Source: CAD feature listing. Evaluate the final solid. Frame: model axes, mm. A direction names the side the tool comes from. Coordinates: 2 decimals unless noted, no trailing zeros. Write each loop counter-clockwise with the first axis right and the second up, starting at its lowest first coordinate (ties: lowest second). Pieces come first, ordered by that corner, then holes. Notation, with made-up numbers: (-31, -22.75) - (-14, -22.75) arc R17 ccw to (-14, -6.75) - close; hole circle Ø11 at (28.5, -25.5). An arc over 180 degrees is marked (long way). One line per item, written item: value.
Autodesk Inventor part; units mm, degrees
ref_plane "YZ Plane" through (0, 0, 0) normal (1, 0, 0) x (0, 1, 0)
ref_plane "XZ Plane" through (0, 0, 0) normal (0, 1, 0) x (-1, 0, 0)
ref_plane "XY Plane" through (0, 0, 0) normal (0, 0, 1) x (1, 0, 0)
sketch "Sketch1" plane through (0, 0, 0) normal (0, 0, 1) x (1, 0, 0)
  arc A0 (6.1342, -1.6415) -> (-4.4197, 4.5595) centre (0, 0) ccw
  circle A1 centre (0, 0) radius 9.525 construction
  line L0 (3.175, -12.7) -> (-22.225, -12.7)
  line L1 (-22.225, -12.7) -> (-22.225, -63.5)
  line L2 (-22.225, -63.5) -> (3.175, -63.5)
  line L3 (3.175, -63.5) -> (3.175, -12.7)
  line L4 (3.175, -12.7) -> (-22.225, -63.5) construction
  line L5 (-22.225, -12.7) -> (3.175, -63.5) construction
  line L6 (9.525, 7.0623) -> (9.525, -12.9681) construction
  circle A2 centre (-9.525, -25.4) radius 2.4892
  circle A3 centre (-9.525, -38.1) radius 2.4892
  circle A4 centre (-9.525, -50.8) radius 2.4892
  circle A5 centre (0, 0) radius 2.3813
  line L7 (3.175, -12.7) -> (6.1342, -1.6415)
  line L8 (-4.4197, 4.5595) -> (-22.225, -12.7)
  line L9 (3.175, -63.5) -> (-22.225, -63.5)
  line L10 (-22.225, -63.5) -> (-22.225, -57.15)
  line L11 (-22.225, -57.15) -> (3.175, -57.15)
  line L12 (3.175, -57.15) -> (3.175, -63.5)
  line L13 (-22.225, -63.5) -> (-13.843, -63.5)
  line L14 (-13.843, -63.5) -> (-13.843, -44.45)
  line L15 (-13.843, -44.45) -> (-22.225, -44.45)
  line L16 (-22.225, -44.45) -> (-22.225, -63.5)
  point P0 (-13.843, -57.15)
  point P1 (3.175, -57.15)
  dimension "d0" = 12.7
  dimension "d1" = 19.05
  dimension "d2" = 25.4
  dimension "d4" = 6.35
  dimension "d5" = 4.9784
  dimension "d8" = 12.7
  dimension "d13" = 4.7625
  dimension "d17" = 3.175
  dimension "d18" = 12.7
  dimension "d19" = 6.35
  dimension "d20" = 8.382
  dimension "d21" = 19.05
extrude "Extrusion1" add sketch "Sketch1" along normal blind 3.175 contours L7 L0 L8 A0 | L3 L11 L14 L15 L1 L0 | L15 L14 L11 L1
fillet "Fillet1" radius 3.175 4 edges at (3.175, -12.7, 1.5875) (-22.225, -12.7, 1.5875) (3.175, -57.15, 1.5875) (-22.225, -57.15, 1.5875)
properties part number "Top Bearing Plate (R4 - 0.25in Between Stages)" material "Aluminum 6061"
1) Material intervals for line 1 (Y direction, x = 0, z = 1.7); line 2 (Y direction, x = -10, z = 0.75); line 3 (Y direction, x = -11, z = 2), sorted ascending.
Values found:
line 1: -57.15 to -2.38, 2.38 to 6.35
line 2: -57.15 to -53.24, -48.36 to -40.54, -35.66 to -27.84, -22.96 to -0.85
line 3: -57.15 to -52.81, -48.79 to -40.11, -36.09 to -27.41, -23.39 to -1.82
2) Contact query for flat-ended pins moving along their axis: P1, Ø4, axis at x = -9.525, y = -50.8, coming from the -Z side; P2, Ø1.6, axis at y = -23.5, z = 1, coming from the +X side (3 decimals). Output: stop coordinate, or through.
Values found:
P1: through
P2: x = 3.175
3) Draft query along Y for faces 3 (the cylindrical face through (2.22, -56.245, 1.61)), 4 (the flat face through (-5, -25, 0)), 5 (the cylindrical face through (-11.36, -27.08, 1.57)), 6 (the cylindrical face through (1.1, 2.11, 1.57)). Return one class per face: released by +Y, released by -Y, zero draft, split by the parting line, or undercut.
Values found:
face 3: released by -Y
face 4: zero draft
face 5: undercut
face 6: undercut
4) Reachability of faces 1 (the flat face through (-12.722, -3.488, 1.565)), 2 (the flat face through (3.175, -34, 2)) from +Z, -Z, +X, -X, +Y, -Y: full face, straight path, thin tool, end or side. Return the list, or none.
Values found:
face 1: +Z, -Z, -X, +Y
face 2: +Z, -Z, +X, -Y
5) Section query C-C on y = -17. Output: boundary loops of the cut face in (x, z) (3 decimals).
Values found:
outline: (-22.225, 0) - (3.175, 0) - (3.175, 3.175) - (-22.225, 3.175) - close
6) Section query A-A on y = -50.8. Output: boundary loops of the cut face in (x, z) (3 decimals).
Values found:
outline: (-22.225, 0) - (-12.014, 0) - (-12.014, 3.175) - (-22.225, 3.175) - close; (-7.036, 0) - (3.175, 0) - (3.175, 3.175) - (-7.036, 3.175) - close
7) Section query B-B on z = 2.2. State how many separate pieces and enclosed holes the cut face has, then the cut area to 3 significant figures.
Values found:
separate pieces: 1
enclosed holes: 4
area: 1,380 mm2
8) Section query D-D on x = -6.25. Output: boundary loops of the cut face in (y, z) (3 decimals).
Values found:
outline: (-57.15, 0) - (2.785, 0) - (2.785, 3.175) - (-57.15, 3.175) - close
